The figure shows three views and two pictorial views of one solid part (mm, origin at its lowest corner). Answer the questions. Round coordinates to 2 decimals unless told otherwise and drop trailing zeros. Write each loop counter-clockwise with the first axis right and the second up, starting at its lowest first coordinate (ties: lowest second). Pieces come first, ordered by that corner, then holes.
Item 1: Find the intervals of material crossed by probe 1 along Z at (x, y) = (54, 1.75) (1 decimal); probe 2 along Z at (x, y) = (34.5, 2) (1 decimal); probe 3 along X at (y, z) = (5.5, 22) (1 decimal), in increasing order.
Item 2: Find section A-A on z = 80. Give the vertices of the cut face in (x, y), then the cut area to 3 significant figures.
Item 3: Find section C-C on z = 50. Give the vertices of the cut face in (x, y).
Item 4: Each of these flat-tipped pins is pushed along its axis until it touches: pin 1 (6 mm diameter, centred on y = 4.5, z = 74.5, fed in from -X); pin 2 (2 mm diameter, centred on x = 40, y = 7, fed in from +Z); pin 3 (5 mm diameter, centred on y = 7, z = 60, fed in from -X) (1 decimal); pin 4 (18 mm diameter, centred on x = 21.47, z = 59.27, fed in from +Y). Where does it stop, or does it pass through?
Item 5: Find section B-B on x = 50. Give the vertices of the cut face in (y, z), then the cut area to 3 significant figures.
Item 6: For a pull along X with two mould halves and no side action, classify the marked faces 1, 2, 3 and 4 as +X half, -X half, draft (parallel to the pull), parting line (faces both ways), or undercut.
Item 7: Find section D-D on y = 8. Give the vertices of the cut face in (x, z), then the cut area to 3 significant figures.
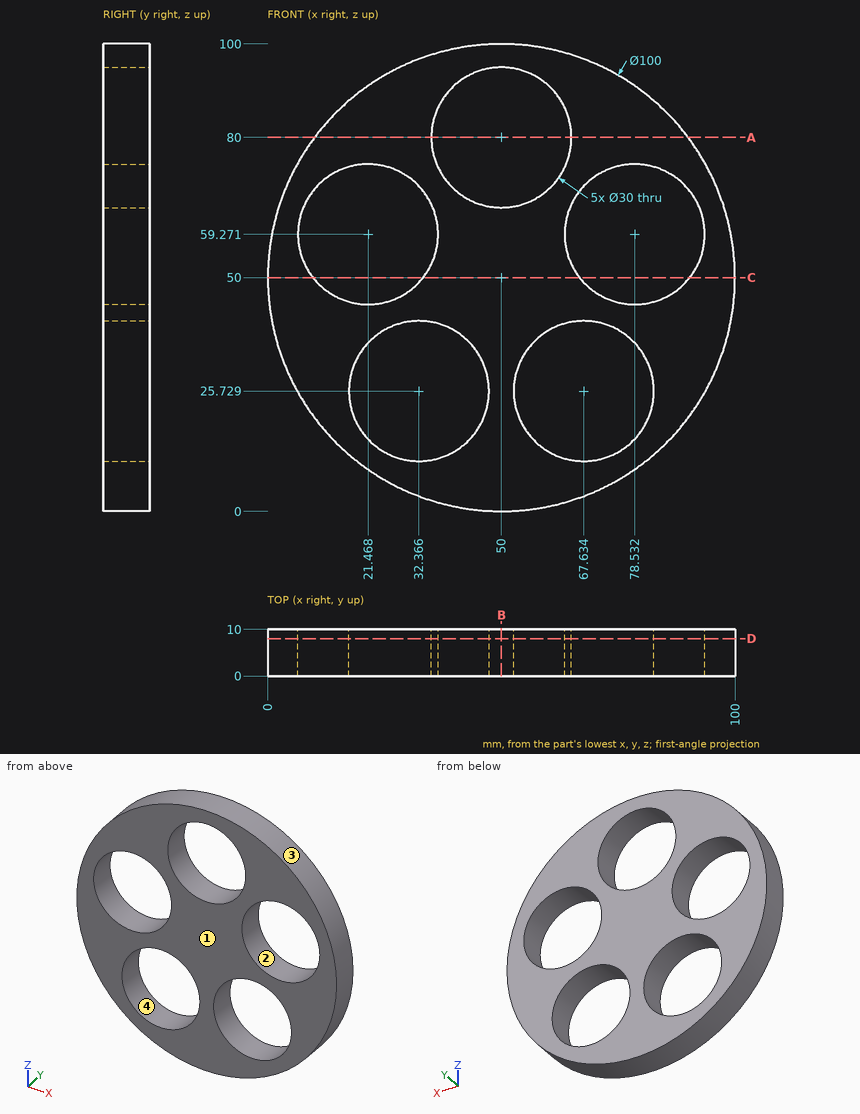
Check values:
1. probe 1: z = 0.2 to 19.5, 32 to 65.5, 94.5 to 99.8
1. probe 2: z = 2.5 to 10.9, 40.6 to 51.8, 66.7 to 97.5
1. probe 3: x = 8.6 to 17.8, 46.9 to 53.1, 82.2 to 91.4
2. outline: (10, 0) - (35, 0) - (35, 10) - (10, 10) - close; (65, 0) - (90, 0) - (90, 10) - (65, 10) - close
2. area: 500 mm2
3. outline: (0, 0) - (9.68, 0) - (9.68, 10) - (0, 10) - close; (33.26, 0) - (66.74, 0) - (66.74, 10) - (33.26, 10) - close; (90.32, 0) - (100, 0) - (100, 10) - (90.32, 10) - close
4. pin 1: stops at x = 4.86
4. pin 2: stops at z = 99.18
4. pin 3: stops at x = 0.6
4. pin 4: passes through
5. outline: (0, 0) - (10, 0) - (10, 65) - (0, 65) - close; (0, 95) - (10, 95) - (10, 100) - (0, 100) - close
5. area: 700 mm2
6. face 1: draft
6. face 2: undercut
6. face 3: parting line
6. face 4: undercut
7. outline: circle Ø100 at (50, 50); hole circle Ø30 at (21.47, 59.27); hole circle Ø30 at (32.37, 25.73); hole circle Ø30 at (50, 80); hole circle Ø30 at (67.63, 25.73); hole circle Ø30 at (78.53, 59.27)
7. area: 4,320 mm2
